from build123d import *

# Parameters (mm, degrees)
BOSS_EXTRUDE1_DEPTH = 5
SKETCH2_W           = 7.25
SKETCH2_H           = 5
BOSS_EXTRUDE2_DEPTH = 65
SKETCH3_W           = 7.25
SKETCH3_H           = 5
BOSS_EXTRUDE3_DEPTH = 65
SKETCH4_W           = 5
SKETCH4_H           = 11.25
BOSS_EXTRUDE4_DEPTH = 51
FILLET2_R           = 1
FILLET3_SIZE        = 3
FILLET3_SIZE_2      = 10


with BuildPart() as part:
    # Sketch1 → Boss-Extrude1 (new body)
    with BuildSketch(Plane(origin=(0, 0, 0), x_dir=(1, 0, 0), z_dir=(0, 1, 0))):
        with BuildLine():
            Line((10, 33), (10, 0))
            ThreePointArc((10, 0), (0, -10), (-10, 0))
            Line((-10, 0), (-10, 33))
            ThreePointArc((-10, 33), (0, 43), (10, 33))
        make_face()
        with BuildLine():
            Line((-3, 0), (-3, 33))
            ThreePointArc((-3, 33), (0, 36), (3, 33))
            Line((3, 33), (3, 0))
            ThreePointArc((3, 0), (0, -3), (-3, 0))
        make_face(mode=Mode.SUBTRACT)
    extrude(amount=BOSS_EXTRUDE1_DEPTH)

    # Sketch2 → Boss-Extrude2 (add)
    with BuildSketch(Plane(origin=(10, 0, 0), x_dir=(0, 0, -1), z_dir=(1, 0, 0))):
        with Locations((16.5, 2.5)):
            Rectangle(SKETCH2_W, SKETCH2_H)
    extrude(amount=BOSS_EXTRUDE2_DEPTH)

    # Sketch3 → Boss-Extrude3 (add)
    with BuildSketch(Plane.ZY.offset(10)):
        with Locations((-16.5, 2.5)):
            Rectangle(SKETCH3_W, SKETCH3_H)
    extrude(amount=BOSS_EXTRUDE3_DEPTH)

    # Sketch4 → Boss-Extrude4 (add)
    with BuildSketch(Plane(origin=(0, 5, 0), x_dir=(1, 0, 0), z_dir=(0, 1, 0))):
        with Locations((72.5, 16.5)):
            Rectangle(SKETCH4_W, SKETCH4_H)
        with Locations((-72.5, 16.5)):
            Rectangle(SKETCH4_W, SKETCH4_H)
    extrude(amount=BOSS_EXTRUDE4_DEPTH)

    # Fillet2
    fillet2_edges = [part.edges().sort_by_distance(p)[0] for p in [
        (72.5, 5, -20.125),
        (72.5, 5, -12.875),
        (-72.5, 5, -12.875),
        (-72.5, 5, -20.125),
    ]]
    fillet(fillet2_edges, radius=FILLET2_R)

    # Fillet3
    # an asymmetric fillet: 10, 3 mm, written as the material it adds along each edge
    with BuildSketch(Plane(origin=(70, 5, -20.125), x_dir=(-1, 0, 0), z_dir=(0, 0, 1))) as fillet3_piece_1:
        with BuildLine():
            Bezier((FILLET3_SIZE, 0), (0, 0), (0, -FILLET3_SIZE_2), weights=[1, 0.707106781, 1])
            Line((0, -FILLET3_SIZE_2), (0, 0))
            Line((0, 0), (FILLET3_SIZE, 0))
        make_face()
    extrude(amount=7.25)
    with BuildSketch(Plane(origin=(-70, 5, -20.125), x_dir=(0, 1, 0), z_dir=(0, 0, 1))) as fillet3_piece_2:
        with BuildLine():
            Bezier((FILLET3_SIZE_2, 0), (0, 0), (0, -FILLET3_SIZE), weights=[1, 0.707106781, 1])
            Line((0, -FILLET3_SIZE), (0, 0))
            Line((0, 0), (FILLET3_SIZE_2, 0))
        make_face()
    extrude(amount=7.25)


solid = part.part
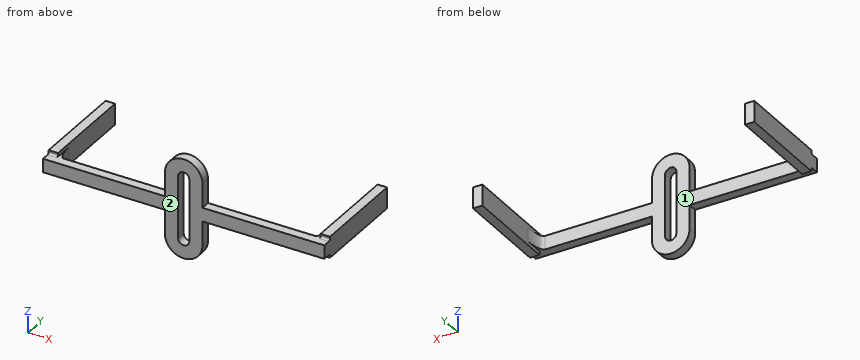
CAD build for the part. Positions are in the model's coordinates, mm. Face numbers are marked on the shaded views. Coordinates: 2 decimals unless noted, no trailing zeros. Write each loop counter-clockwise with the first axis right and the second up, starting at its lowest first coordinate (ties: lowest second). Pieces come first, ordered by that corner, then holes. Notation, with made-up numbers: M 11,26.25 L 27,26.25 A19 cw 27,58.25 Z; hole C 31,24 d1. An arc over 180 degrees is marked long. Answer as a JSON object with one key per item and string values. Group by question number.
1) Mould opens along X. For the marked faces 1 and 2 say: +X half, -X half, draft (parallel to the pull), parting line (faces both ways), or undercut.
2) Saw through at B-B (x = 0). Write the cut outline in (y, z), plus the area to 3 significant figures.
3) Pin check, flat tips, straight feed: pin 1 Ø4 at (x, y) = (-72.5, 18) entering from +Z (3 decimals); pin 2 Ø1.5 at (x, y) = (-73, 42.5) entering from -Z (3 decimals); pin 3 Ø5.5 at (y, z) = (3, -4.5) entering from +X. Stop position of each tip, or through.
4) Saw through at D-D (z = -38.5). Write the cut outline in (x, y), plus the area to 3 significant figures.
5) Saw through at C-C (x = 34.5). Write the cut outline in (y, z) (3 decimals).
6) Wall check: line 1 (X direction, y = 29.5, z = -12); line 2 (Y direction, x = -43.5, z = -15); line 3 (Z direction, x = 35, y = 4) (3 decimals). Give the ranges that are in metal, low to high. Write a range as from..to.
7) Saw through at A-A (z = -31). Write the cut outline in (x, y).
Values follow:
{
 "1": {"face 1": "undercut", "face 2": "draft"},
 "2": {"outline": "M 0,-43 L 5,-43 L 5,-36 L 0,-36 Z; M 0,3 L 5,3 L 5,10 L 0,10 Z", "area": "70.0 mm2"},
 "3": {"pin 1": "stops at z = -10.875", "pin 2": "stops at z = -22.125", "pin 3": "stops at x = 10"},
 "4": {"outline": "M -8.35,0 L 8.35,0 L 8.35,5 L -8.35,5 Z", "area": "83.5 mm2"},
 "5": {"outline": "M 0,-20.125 L 5,-20.125 L 5,-12.875 L 0,-12.875 Z"},
 "6": {"line 1": "x = -75..-70, 70..75", "line 2": "y = 0..5", "line 3": "z = -20.125..-12.875"},
 "7": {"outline": "M -10,0 L -3,0 L -3,5 L -10,5 Z; M 3,0 L 10,0 L 10,5 L 3,5 Z"}
}
